from build123d import *

# Parameters (mm, degrees)
SKETCH_R     = 15
PAD_DEPTH    = 7
SKETCH001_R  = 16
PAD001_DEPTH = 1
SKETCH002_R  = 16
PAD002_DEPTH = 1
SKETCH003_R  = 2.6
POCKET_DEPTH = 9.001


with BuildPart() as part:
    # Sketch → Pad (new body)
    with BuildSketch(Plane.XY):
        Circle(SKETCH_R)
    extrude(amount=PAD_DEPTH)

    # Sketch001 (on Face3 of Pad) → Pad001 (join)
    with BuildSketch(Plane.XY.offset(7)):
        Circle(SKETCH001_R)
    extrude(amount=PAD001_DEPTH)

    # Sketch002 (on Face2 of Pad001) → Pad002 (join)
    with BuildSketch(Plane(origin=(0, 0, 0), x_dir=(1, 0, 0), z_dir=(0, 0, -1))):
        Circle(SKETCH002_R)
    extrude(amount=PAD002_DEPTH)

    # Sketch003 (on Face6 of Pad002) → Pocket (cut, through all)
    with BuildSketch(Plane(origin=(0, 0, -1), x_dir=(1, 0, 0), z_dir=(0, 0, -1))):
        Circle(SKETCH003_R)
    extrude(amount=-POCKET_DEPTH, mode=Mode.SUBTRACT)


solid = part.part
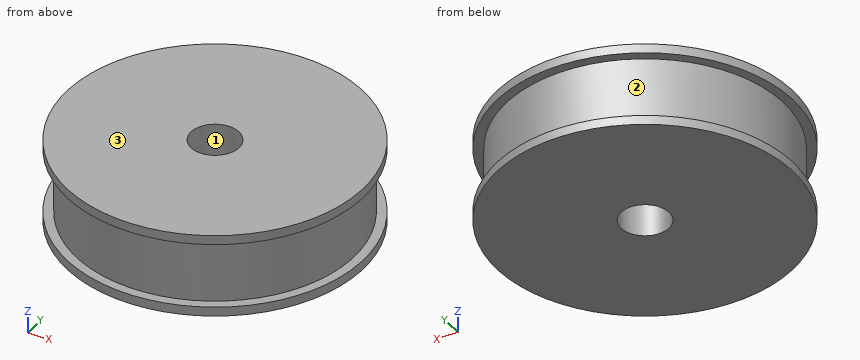
Can you work these out from the model? Positions are in its coordinate system, mm. Face numbers are marked on the shaded views. Give positions to 0.01 mm unless a question says otherwise; leave off trailing zeros. Write each loop counter-clockwise with the first axis right and the second up, starting at its lowest first coordinate (ties: lowest second). Pieces come first, ordered by that corner, then holes. Notation, with made-up numbers: (-11.75, 23.5) -> (-4.75, 23.5) arc R10 ccw to (-4.75, 40.5) -> close; hole circle Ø3 at (-9, -18.5). An arc over 180 degrees is marked (long way). Answer as a JSON object with one key per item and string values. Group by question number.
Item 1: We'd pull the mould along Y, two halves only. Please class the marked faces 1, 2 and 3: +Y half, -Y half, draft (parallel to the pull), parting line (faces both ways), or undercut.
Item 2: Please list where these lines run through material, in increasing order: line 1 (Y direction, x = 0, z = 2.75); line 2 (Z direction, x = 9, y = -12.5); line 3 (X direction, y = -1.5, z = 2.5). Write a range as [from, to].
Item 3: Suppose I cut it at D-D (y = -14). Please give me the cut outline in (x, z).
Item 4: Suppose I cut it at A-A (x = 0). Please give me the cut outline in (y, z), plus the area to 3 significant figures.
Item 5: Suppose I cut it at C-C (z = 6.5). Please give me the cut outline in (x, y).
Item 6: I'm going to push flat-ended pins straight in: P1, Ø1, axis at y = 2, z = 4, coming from the +X side; P2, Ø4.5, axis at x = 0, y = 0, coming from the -Z side; P3, Ø1, axis at x = 9, z = 2, coming from the +Y side; P4, Ø1.5, axis at x = 10.5, z = 5.5, coming from the +Y side. Where does each tip first touch, or does it pass through?
Findings:
{
 "1": {"face 1": "undercut", "face 2": "parting line", "face 3": "draft"},
 "2": {"line 1": "y = [-15, -2.6], [2.6, 15]", "line 2": "z = [-1, 0], [7, 8]", "line 3": "x = [-14.92, -2.12], [2.12, 14.92]"},
 "3": {"outline": "(-7.75, -1) -> (7.75, -1) -> (7.75, 0) -> (5.39, 0) -> (5.39, 7) -> (7.75, 7) -> (7.75, 8) -> (-7.75, 8) -> (-7.75, 7) -> (-5.39, 7) -> (-5.39, 0) -> (-7.75, 0) -> close"},
 "4": {"outline": "(-16, -1) -> (-2.6, -1) -> (-2.6, 8) -> (-16, 8) -> (-16, 7) -> (-15, 7) -> (-15, 0) -> (-16, 0) -> close; (2.6, -1) -> (16, -1) -> (16, 0) -> (15, 0) -> (15, 7) -> (16, 7) -> (16, 8) -> (2.6, 8) -> close", "area": "227 mm²"},
 "5": {"outline": "circle Ø30 at (0, 0); hole circle Ø5.2 at (0, 0)"},
 "6": {"P1": "stops at x = 14.92", "P2": "passes through", "P3": "stops at y = 12.36", "P4": "stops at y = 11.4"}
}
